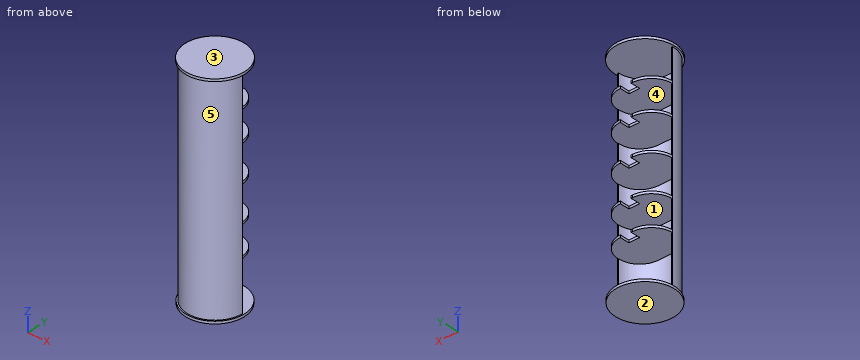
from build123d import *

# Parameters (mm, degrees)
BOSS_EXTRUDE1_DEPTH = 2
LPATTERN1_COUNT     = 2
LPATTERN1_PITCH     = 25
SKETCH7_R           = 24.15
BOSS_EXTRUDE4_DEPTH = 2
LPATTERN2_COUNT     = 3
LPATTERN2_PITCH     = 30
LPATTERN3_START     = 110
LPATTERN3_DEPTH     = 2
SKETCH10_R          = 24.446416427
BOSS_EXTRUDE6_DEPTH = 2
BOSS_EXTRUDE8_DEPTH = 177
CUT_EXTRUDE1_START  = -2
CUT_EXTRUDE1_DEPTH  = 112


# Read off the part's stored shape, not the designer's step: LPattern3
with BuildPart() as part:
    # Sketch2 → Boss-Extrude1 (new body)
    with BuildSketch(Plane.XY):
        with BuildLine():
            Line((-28.088306633, 28.685216936), (-18.088252628, 28.667649742))
            ThreePointArc((-18.088252628, 28.667649742), (-0.619022007, 11.136934368), (-18.14973738, -6.332296253))
            Line((-18.14973738, -6.332296253), (-28.149791386, -6.314729058))
            ThreePointArc((-28.149791386, -6.314729058), (-45.619022007, 11.215986315), (-28.088306633, 28.685216936))
        make_face()
    extrude(amount=BOSS_EXTRUDE1_DEPTH)


with BuildPart() as lpattern1_1:
    # LPattern1: pattern copy
    add(part.part.moved(Location(Vector(0, 0, 1) * (1 * LPATTERN1_PITCH))))


with BuildPart() as body_3:
    # Sketch7 → Boss-Extrude4 (new body)
    with BuildSketch(Plane.XY.offset(-40)):
        with Locations((-22.885176255, 11.436449293)):
            Circle(SKETCH7_R)
    extrude(amount=-BOSS_EXTRUDE4_DEPTH)


with BuildPart() as lpattern2_1:
    # LPattern2: pattern copy
    add(lpattern1_1.part.moved(Location(Vector(0, 0, 1) * (1 * LPATTERN2_PITCH))))


with BuildPart() as lpattern2_2:
    # LPattern2: pattern copy
    add(lpattern1_1.part.moved(Location(Vector(0, 0, 1) * (2 * LPATTERN2_PITCH))))


with BuildPart() as body_6:
    # LPattern3 outline → LPattern3 (new body)
    with BuildSketch(Plane.XY.offset(LPATTERN3_START)):
        with BuildLine():
            ThreePointArc((-28.088306633, 28.685216936), (-45.619022007, 11.215986316), (-28.149791386, -6.314729058))
            Line((-28.149791386, -6.314729058), (-18.14973738, -6.332296253))
            ThreePointArc((-18.14973738, -6.332296253), (-0.619022007, 11.136934369), (-18.088252628, 28.667649742))
            Line((-18.088252628, 28.667649742), (-28.088306633, 28.685216936))
        make_face()
    extrude(amount=LPATTERN3_DEPTH)


with BuildPart() as body_7:
    # Sketch10 → Boss-Extrude6 (new body)
    with BuildSketch(Plane.XY.offset(137)):
        with Locations((-22.885176255, 11.436449293)):
            Circle(SKETCH10_R)
    extrude(amount=BOSS_EXTRUDE6_DEPTH)


with BuildPart() as part_1:
    add(part.part)

    add(lpattern1_1.part)  # Boss-Extrude8 merges LPattern1_1

    add(body_3.part)  # Boss-Extrude8 merges body 3

    add(lpattern2_1.part)  # Boss-Extrude8 merges LPattern2_1

    add(lpattern2_2.part)  # Boss-Extrude8 merges LPattern2_2

    add(body_6.part)  # Boss-Extrude8 merges body 6

    add(body_7.part)  # Boss-Extrude8 merges body 7
    # Sketch8 → Boss-Extrude8 (add)
    with BuildSketch(Plane.XY.offset(-40)):
        with BuildLine():
            Line((-45.885176255, 11.436449293), (-44.885176255, 11.436449293))
            ThreePointArc((-44.885176255, 11.436449293), (-22.885176255, -10.563550707), (-0.885176255, 11.436449293))
            Line((-0.885176255, 11.436449293), (0.114823745, 11.436449293))
            ThreePointArc((0.114823745, 11.436449293), (-22.885176255, -11.563550707), (-45.885176255, 11.436449293))
        make_face()
    extrude(amount=BOSS_EXTRUDE8_DEPTH)

    # Sketch12 → Cut-Extrude1 (cut)
    with BuildSketch(Plane.XY.offset(2).offset(CUT_EXTRUDE1_START)):
        Polygon((-26.739417039, 28.682847328), (-17.739430926, 28.667036963), (-17.753484584, 20.667049308), (-26.753470697, 20.682859673), align=None)
    extrude(amount=CUT_EXTRUDE1_DEPTH, mode=Mode.SUBTRACT)


solid = part_1.part
For this review, take the finished solid that the model builds, in its own axes (mm). Face numbers are marked on the shaded views. A direction names the side the tool comes from. Coordinates: 2 decimals unless noted, no trailing zeros. Order: outer loops, then holes, each group sorted by start corner. A loop starts at its lowest first (then second) coordinate and runs counter-clockwise, first axis right, second up. Notation, with made-up numbers: (-4, 26.5) -> (33, 26.5) arc R24 ccw to (33, 36.5) -> close; hole circle Ø2 at (30.25, -18). An arc over 180 degrees is marked (long way). Return JSON: item names as keys, results as strings.
1. We need section C-C on z = 62. Write out the cut boundary in (x, y).
Answer block:
{"outline": "(-45.89, 11.44) arc R23 ccw to (0.11, 11.44) -> (-0.89, 11.44) arc R22 cw to (-44.89, 11.44) -> close"}
2. For pin 1 Ø12 at (x, z) = (-10, 14.5) entering from +Y; pin 2 Ø4 at (x, z) = (-28, 46) entering from +Y; pin 3 Ø8 at (y, z) = (-3.5, 64.5) entering from +X, all flat-tipped, find the tip position at first contact; note any pin that passes through.
Answer block:
{"pin 1": "y = 0.15", "pin 2": "y = -9.38", "pin 3": "x = -2.65"}
3. The part is to be moulded in two halves that separate along X. For the marked faces 3, 4 and 5, say which applies: +X half, -X half, draft (parallel to the pull), parting line (faces both ways), or undercut.
Answer block:
{"face 3": "draft", "face 4": "undercut", "face 5": "parting line"}
4. We need section B-B on y = 18.5. Write out the cut boundary in (x, z), and give its area (3 significant figures).
Answer block:
{"outline": "(-46.29, 137) -> (0.52, 137) -> (0.52, 139) -> (-46.29, 139) -> close; (-45.98, -42) -> (0.21, -42) -> (0.21, -40) -> (-45.98, -40) -> close; (-44.02, 0) -> (-2.23, 0) -> (-2.23, 2) -> (-44.02, 2) -> close; (-44.02, 25) -> (-2.23, 25) -> (-2.23, 27) -> (-44.02, 27) -> close; (-44.02, 55) -> (-2.23, 55) -> (-2.23, 57) -> (-44.02, 57) -> close; (-44.02, 85) -> (-2.23, 85) -> (-2.23, 87) -> (-44.02, 87) -> close; (-44.02, 110) -> (-2.23, 110) -> (-2.23, 112) -> (-44.02, 112) -> close", "area": "604 mm²"}
5. For line 1 (Z direction, x = -19, y = 29); line 2 (X direction, y = 4, z = -34); line 3 (Y direction, x = -22, z = -7), list the stretches that pass through material, from the lowest coordinate up. Write a range as from..to.
Answer block:
{"line 1": "-42..-40, 137..139", "line 2": "-44.65..-43.59, -2.18..-1.12", "line 3": "-11.55..-10.55"}
6. Machinability: for the marked faces 1 and 2, which of the approach directions +Z, -Z, +X, -X, +Y, -Y give a long, thin tool a straight path to every point of the face, cutting with its end or side? Answer none if there is none.
Answer block:
{"face 1": "+Y", "face 2": "-Z, +X, -X, +Y, -Y"}
7. We need section A-A on x = -31. State how many separate pieces and enclosed holes the cut face has, and give its area (3 significant figures).
Answer block:
{"separate pieces": "6", "enclosed holes": "0", "area": "718 mm²"}
